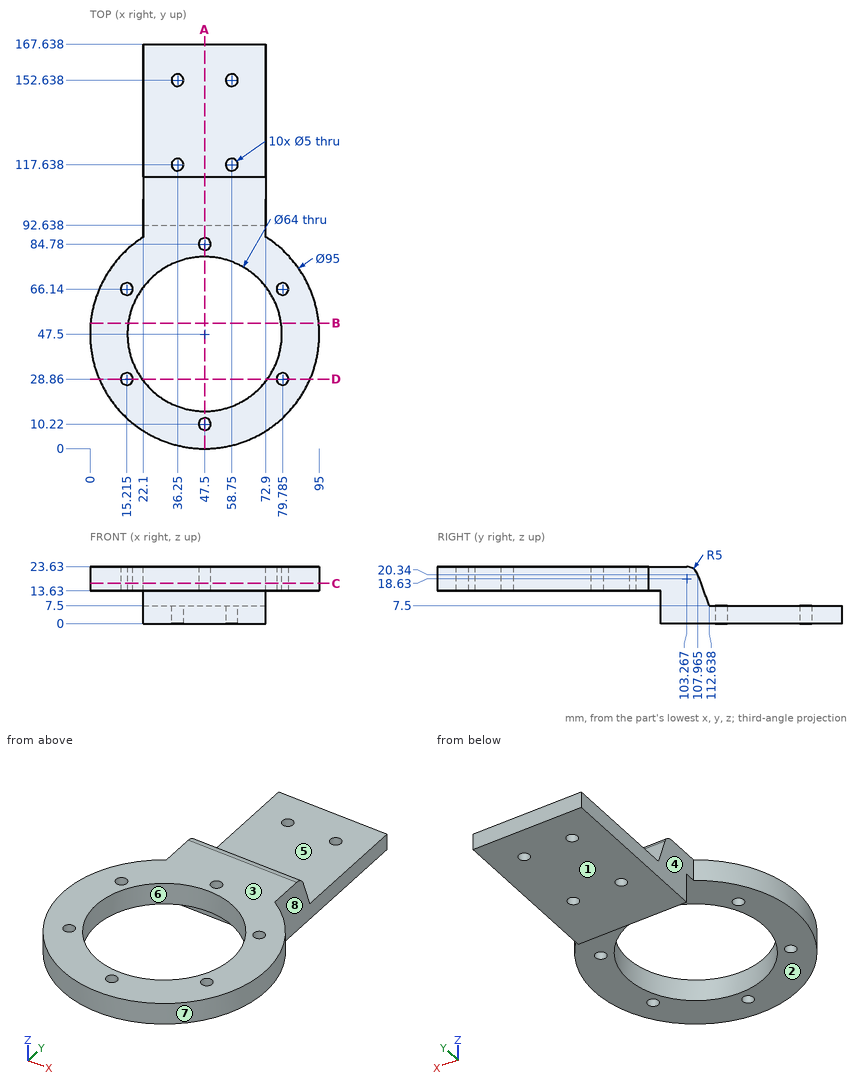
Study the drawing (mm; zero at the part's minimum x, y, z) and answer. A direction names the side the tool comes from. Give positions to 0.01 mm unless a question says otherwise; leave off trailing zeros. Write each loop counter-clockwise with the first axis right and the second up, starting at its lowest first coordinate (ties: lowest second). Pieces come first, ordered by that corner, then holes.
Item 1: Section B-B, the plane y = 52 is taken. Write down the section's boundary in (x, z), plus the area to 3 significant figures.
Item 2: Which of the six approach directions +Z, -Z, +X, -X, +Y, -Y give full straight-line access (tool end or side, diameter ignored) to the marked faces 1, 2, 3, 4 and 5?
Item 3: Flat-ended cylindrical pins translate along their axes: P1, Ø12, axis at x = 77.5, y = 77.5, coming from the -Z side; P2, Ø3, axis at x = 68.5, z = 7, coming from the -Y side; P3, Ø4.5, axis at x = 15.21, y = 66.14, coming from the +Z side; P4, Ø12, axis at x = 33, z = 11, coming from the -Y side. Find the tip coordinate at first contact, or state that the pin passes through.
Item 4: Section C-C, the plane z = 16.75 is taken. Write down the section's boundary in (x, y) (1 decimal), plus the area to 3 significant figures.
Item 5: Determine the mould class of the marked faces 6, 7 and 8 for opening direction X: released by +X, released by -X, zero draft, split by the parting line, or undercut.
Item 6: Section A-A, the plane x = 47.5 is taken. Write down the section's boundary in (y, z) (1 decimal), plus the area to 3 significant figures.
Item 7: Find the intervals of material crossed by line 1 along Y through (x, z) = (58.75, 2.75); line 2 along X through (y, z) = (93, 1.5); line 3 along Z through (x, y) = (78, 35), in increasing order.
Item 8: Section D-D, the plane y = 28.86 is taken. Write down the section's boundary in (x, z) (1 decimal).
Completed:
1. outline: (0.21, 13.63) - (15.82, 13.63) - (15.82, 23.63) - (0.21, 23.63) - close; (79.18, 13.63) - (94.79, 13.63) - (94.79, 23.63) - (79.18, 23.63) - close
1. area: 312 mm2
2. face 1: -Z, +X, -X, +Y, -Y
2. face 2: -Z, +X, -X, -Y
2. face 3: +Z, +X, -X, +Y, -Y
2. face 4: +Z, -Z, -X, +Y
2. face 5: +Z, +X, -X, +Y
3. P1: stops at z = 13.63
3. P2: stops at y = 92.64
3. P3: passes through
3. P4: stops at y = 0.88
4. outline: (22.1, 87.6) arc R47.5 ccw (long way) to (72.9, 87.6) - (72.9, 109.3) - (22.1, 109.3) - close; hole circle Ø5 at (15.2, 28.9); hole circle Ø5 at (15.2, 66.1); hole circle Ø64 at (47.5, 47.5); hole circle Ø5 at (47.5, 10.2); hole circle Ø5 at (47.5, 84.8); hole circle Ø5 at (79.8, 28.9); hole circle Ø5 at (79.8, 66.1)
4. area: 4,600 mm2
5. face 6: undercut
5. face 7: split by the parting line
5. face 8: released by +X
6. outline: (0, 13.6) - (7.7, 13.6) - (7.7, 23.6) - (0, 23.6) - close; (12.7, 13.6) - (15.5, 13.6) - (15.5, 23.6) - (12.7, 23.6) - close; (79.5, 13.6) - (82.3, 13.6) - (82.3, 23.6) - (79.5, 23.6) - close; (87.3, 13.6) - (92.6, 13.6) - (92.6, 0) - (167.6, 0) - (167.6, 7.5) - (112.6, 7.5) - (108, 20.3) arc R5 ccw to (103.3, 23.6) - (87.3, 23.6) - close
6. area: 1,020 mm2
7. line 1: y = 92.64 to 115.14, 120.14 to 150.14, 155.14 to 167.64
7. line 2: x = 22.1 to 72.9
7. line 3: z = 13.63 to 23.63
8. outline: (3.8, 13.6) - (12.7, 13.6) - (12.7, 23.6) - (3.8, 23.6) - close; (17.7, 13.6) - (21.5, 13.6) - (21.5, 23.6) - (17.7, 23.6) - close; (73.5, 13.6) - (77.3, 13.6) - (77.3, 23.6) - (73.5, 23.6) - close; (82.3, 13.6) - (91.2, 13.6) - (91.2, 23.6) - (82.3, 23.6) - close
